The listing builds one solid part. Answer for the finished solid, in the listing's coordinates (mm). A direction names the side the tool comes from. Coordinates: 2 decimals unless noted, no trailing zeros. Order: outer loops, then holes, each group sorted by start corner. A loop starts at its lowest first (then second) coordinate and runs counter-clockwise, first axis right, second up. Notation, with made-up numbers: (4.25, 8) - (27.25, 8) arc R11 cw to (27.25, 15) - close; hole circle Ø1 at (77, 11.5). An arc over 180 degrees is marked (long way). One line per item, written item: value. Start each with the question number.
Autodesk Inventor part; units mm, degrees
ref_plane "YZ Plane" through (0, 0, 0) normal (1, 0, 0) x (0, 1, 0)
ref_plane "XZ Plane" through (0, 0, 0) normal (0, 1, 0) x (-1, 0, 0)
ref_plane "XY Plane" through (0, 0, 0) normal (0, 0, 1) x (1, 0, 0)
sketch "Sketch1" plane through (0, 0, 0) normal (0, 1, 0) x (-1, 0, 0)
  line L0 (9, 0) -> (45, 0)
  line L1 (54, -9) -> (54, -46.8)
  line L2 (28.8, -72) -> (8.1, -72)
  line L3 (0, -63.9) -> (0, -9)
  arc A0 (54, -9) -> (45, 0) centre (45, -9) ccw
  arc A1 (9, 0) -> (0, -9) centre (9, -9) ccw
  arc A2 (0, -63.9) -> (8.1, -72) centre (8.1, -63.9) ccw
  line L4 (54, -46.8) -> (28.8, -72)
  circle A3 centre (38.233, -36.5794) radius 6
  circle A4 centre (13.039, -61.766) radius 6
  line L5 (44.015, -8.55) -> (8.815, -8.55)
  line L6 (8.815, -8.55) -> (8.815, -17.9)
  line L7 (8.815, -17.9) -> (44.015, -17.9)
  line L8 (44.015, -17.9) -> (44.015, -8.55)
  point P0 (0, 0)
  point P1 (54, -72)
  point P2 (54, 0)
  point P3 (0, -72)
  dimension "d2" = 9
  dimension "d3" = 8.1
  dimension "d7" = 20.7
  dimension "d8" = 36
  dimension "d9" = 37.8
  dimension "d10" = 9
  dimension "d11" = 54.9
  dimension "d12" = 12
  dimension "d13" = 12
  dimension "d14" = 15.767
  dimension "d15" = 18.376
  dimension "d16" = 10.234
  dimension "d17" = 13.039
  dimension "d18" = 38.233
  dimension "d19" = 9.35
  dimension "d20" = 35.2
  dimension "d21" = 8.55
  dimension "d22" = 8.815
  dimension "d23" = 9.985
  dimension "d26" = 23.6245
extrude "Extrusion1" add sketch "Sketch1" along normal blind 9
properties part number "Hip"
(1) Consider probe 1 along X at (y, z) = (7.25, -10.5) (3 decimals); probe 2 along Z at (x, y) = (-22, 2.75); probe 3 along Z at (x, y) = (-39, 3.75). Determine where each line is inside the solid, lowest interval first.
(2) A flat-ended cylindrical pin translates along its axis: pin 1 Ø3 at (x, y) = (-40.5, 7.5) entering from -Z. Find the tip coordinate at first contact, or state that the pin passes through.
(3) The part is cut by section C-C on x = -37.5. Determine the outline of the cut face in (y, z), plus the area to 3 significant figures.
(4) The part is cut by section A-A on z = -16.5. Determine the outline of the cut face in (x, y) (3 decimals).
(5) For faces 1 (the face through (0, 4, -37)), 2 (the face through (-26, 4, -17.9)), determine the directions among +Z, -Z, +X, -X, +Y, -Y from which every point of the face is accessible in a straight line to the end or side of a thin tool.
(6) The part is cut by section B-B on x = -20. Determine the outline of the cut face in (y, z), plus the area to 3 significant figures.
(7) For a pull along X with two mould halves and no side action, classify faces 3 (the face through (-27, 4, 0)), 4 (the face through (-54, 4, -28)), 5 (the face through (-16.26, 4.44, -66.83)) as pulls with the +X half, pulls with the -X half, needs draft (parallel to the pull), parting line crosses it, or undercut.
(8) The part is cut by section D-D on y = 5.25. Determine the outline of the cut face in (x, z) (3 decimals).
Completed:
1. probe 1: x = -54 to -44.015, -8.815 to 0
1. probe 2: z = -72 to -17.9, -8.55 to 0
1. probe 3: z = -61.8 to -42.53, -30.63 to -17.9, -8.55 to 0
2. pin 1: stops at z = -61.8
3. outline: (0, -63.3) - (9, -63.3) - (9, -42.53) - (0, -42.53) - close; (0, -30.62) - (9, -30.62) - (9, -17.9) - (0, -17.9) - close; (0, -8.55) - (9, -8.55) - (9, 0) - (0, 0) - close
3. area: 378 mm2
4. outline: (-54, 0) - (-44.015, 0) - (-44.015, 9) - (-54, 9) - close; (-8.815, 0) - (0, 0) - (0, 9) - (-8.815, 9) - close
5. face 1: +Z, -Z, +X, +Y, -Y
5. face 2: +Y, -Y
6. outline: (0, -72) - (9, -72) - (9, -17.9) - (0, -17.9) - close; (0, -8.55) - (9, -8.55) - (9, 0) - (0, 0) - close
6. area: 564 mm2
7. face 3: needs draft
7. face 4: pulls with the -X half
7. face 5: undercut
8. outline: (-54, -46.8) - (-28.8, -72) - (-8.1, -72) arc R8.1 ccw to (0, -63.9) - (0, -9) arc R9 ccw to (-9, 0) - (-45, 0) arc R9 ccw to (-54, -9) - close; hole circle Ø12 at (-38.233, -36.579); hole (-44.015, -17.9) - (-8.815, -17.9) - (-8.815, -8.55) - (-44.015, -8.55) - close; hole circle Ø12 at (-13.039, -61.766)
